Build history of the part. All positions in model axes, mm. Face numbers are marked on the shaded views. A direction names the side the tool comes from. Coordinates: 2 decimals unless noted, no trailing zeros. Loops run counter-clockwise (first coordinate to the right, second up) from the corner with the lowest first, then second, coordinate; pieces in that order, holes last.
(1) Slice it at A-A (y = 8). Give the cut face in (x, z).
(2) Slice it at D-D (z = 12.5). Give the number of separate pieces and of enclosed holes in the cut face, and give its area (3 significant figures).
(3) Wall check: L1, parallel to Y at x = -55, z = 11.75; L2, parallel to X at y = -48.5, z = 11.25; L3, parallel to X at y = 21.5, z = 11.75. Give the ranges that are in metal, low to high.
(4) Tool access for the marked faces 1 and 2: list every direction of +Z, -Z, +X, -X, +Y, -Y with a clear straight run to the whole face (end or side of a thin tool).
(5) Slice it at C-C (z = 18). Give the cut face in (x, y), and give its area (3 significant figures).
(6) Flat gauge pins, fed straight in: P1, Ø1.5, axis at y = 52.5, z = 7.5, coming from the -X side; P2, Ø1, axis at x = -56, y = -9, coming from the +Z side; P3, Ø3.5, axis at x = -89, z = 8.5, coming from the +Y side; P4, Ø4, axis at x = -59.61, y = -2.83, coming from the +Z side. Where does each tip first touch, or does it go through?
(7) Slice it at B-B (x = -77). Give the cut face in (y, z), and give its area (3 significant figures).
(8) Two-plate mould, pull along X, no slides. Class the marked faces 3, 4, 5 and 6: pulls with the +X half, pulls with the -X half, needs draft (parallel to the pull), parting line crosses it, or undercut.
from build123d import *

# Parameters (mm, degrees)
SALIENTE_EXTRUIR1_DEPTH      = 50
CROQUIS2_W                   = 40
CROQUIS2_H                   = 50
SALIENTE_EXTRUIR2_DEPTH      = 60
SALIENTE_EXTRUIR2_DEPTH_BACK = 31
REDONDEO1_R                  = 10
REDONDEO2_R                  = 10
CORTAR_EXTRUIR2_DEPTH        = 76
REDONDEO6_R                  = 5
VACIADO2_T                   = -3
CROQUIS4_R                   = 5
SALIENTE_EXTRUIR3_DEPTH      = 7
CROQUIS5_R                   = 2.5
CORTAR_EXTRUIR3_DEPTH        = 11
SALIENTE_EXTRUIR4_DEPTH      = 5
CROQUIS6_4_R                 = 2.5
CORTAR_EXTRUIR4_DEPTH        = 21
CORTAR_EXTRUIR7_REACH        = 62
CROQUIS8_R                   = 3.75
CORTAR_EXTRUIR8_REACH        = 64.5
CROQUIS9_W                   = 4
CROQUIS9_H                   = 8
CORTAR_EXTRUIR9_REACH        = 122
CROQUIS10_W                  = 10
CROQUIS10_H                  = 4


with BuildPart() as part:
    # Croquis1 → Saliente-Extruir1 (new body)
    with BuildSketch(Plane.XY):
        with BuildLine():
            Line((-80.606796451, 54.173553719), (-40.606796451, 54.173553719))
            ThreePointArc((-40.606796451, 54.173553719), (-33.53572864, 51.244621531), (-30.606796451, 44.173553719))
            Line((-30.606796451, 44.173553719), (-30.606796451, 4.173553719))
            ThreePointArc((-30.606796451, 4.173553719), (-33.53572864, -2.897514093), (-40.606796451, -5.826446281))
            Line((-40.606796451, -5.826446281), (-80.606796451, -5.826446281))
            ThreePointArc((-80.606796451, -5.826446281), (-87.677864263, -2.897514093), (-90.606796451, 4.173553719))
            Line((-90.606796451, 4.173553719), (-90.606796451, 44.173553719))
            ThreePointArc((-90.606796451, 44.173553719), (-87.677864263, 51.244621531), (-80.606796451, 54.173553719))
        make_face()
    extrude(amount=SALIENTE_EXTRUIR1_DEPTH)

    # Croquis2 → Saliente-Extruir2 (add, two sides)
    with BuildSketch(Plane.XZ.offset(5.826446281)) as saliente_extruir2_sk:
        with Locations((-50.606796451, 25)):
            Rectangle(CROQUIS2_W, CROQUIS2_H)
    extrude(amount=SALIENTE_EXTRUIR2_DEPTH)
    extrude(saliente_extruir2_sk.sketch, amount=-SALIENTE_EXTRUIR2_DEPTH_BACK)

    # Redondeo1
    redondeo1_edges = [part.edges().sort_by_distance(p)[0] for p in [
        (-30.606796451, -65.826446281, 25),
    ]]
    fillet(redondeo1_edges, radius=REDONDEO1_R)

    # Redondeo2
    redondeo2_edges = [part.edges().sort_by_distance(p)[0] for p in [
        (-70.606796451, -65.826446281, 25),
    ]]
    fillet(redondeo2_edges, radius=REDONDEO2_R)

    # Croquis3 → Cortar-Extruir2 (cut)
    with BuildSketch(Plane(origin=(-30.606796451, 0, 0), x_dir=(0, 0, -1), z_dir=(1, 0, 0))):
        Polygon((-20, -55.826446281), (-20, 57.222275959), (-50, 57.222275959), (-50, -55.826446281), (-50, -71.304791729), (-20, -71.304791729), align=None)
    extrude(amount=-CORTAR_EXTRUIR2_DEPTH, mode=Mode.SUBTRACT)

    # Redondeo6
    redondeo6_edges = [part.edges().sort_by_distance(p)[0] for p in [
        (-70.606796451, -5.826446281, 10),
    ]]
    fillet(redondeo6_edges, radius=REDONDEO6_R)

    # Vaciado2
    vaciado2_openings = [part.faces().sort_by_distance(p)[0] for p in [
        (-63.60975761, -5.496074106, 20),
    ]]
    offset(amount=VACIADO2_T, openings=vaciado2_openings, kind=Kind.INTERSECTION)

    # Croquis4 → Saliente-Extruir3 (add)
    with BuildSketch(Plane.XY.offset(3)):
        with Locations((-39.606796451, -2.826446281)):
            Circle(CROQUIS4_R)
        with Locations((-59.606796451, -2.826446281)):
            Circle(CROQUIS4_R)
    extrude(amount=SALIENTE_EXTRUIR3_DEPTH)

    # Croquis5 → Cortar-Extruir3 (cut, through all)
    with BuildSketch(Plane.XY.offset(10)):
        with Locations((-59.606796451, -2.826446281)):
            Circle(CROQUIS5_R)
        with Locations((-39.606796451, -2.826446281)):
            Circle(CROQUIS5_R)
    extrude(amount=-CORTAR_EXTRUIR3_DEPTH, mode=Mode.SUBTRACT)

    # Croquis6 → Saliente-Extruir4 (add)
    with BuildSketch(Plane.XY.offset(20)):
        with BuildLine():
            Line((-35.560225021, 61.520617947), (-48.606796451, 54.173553719))
            Line((-48.606796451, 54.173553719), (-40.606796451, 54.173553719))
            ThreePointArc((-40.606796451, 54.173553719), (-33.53572864, 51.244621531), (-30.606796451, 44.173553719))
            Line((-30.606796451, 44.173553719), (-30.606796451, 36.173553719))
            Line((-30.606796451, 36.173553719), (-28.142904197, 56.564123399))
            ThreePointArc((-28.142904197, 56.564123399), (-30.328790596, 61.321179473), (-35.560225021, 61.520617947))
        make_face()
    extrude(amount=-SALIENTE_EXTRUIR4_DEPTH)

    # Croquis6_4 → Cortar-Extruir4 (cut, through all)
    with BuildSketch(Plane.XY.offset(20)):
        with Locations((-33.106796451, 57.163934776)):
            Circle(CROQUIS6_4_R)
    extrude(amount=-CORTAR_EXTRUIR4_DEPTH, mode=Mode.SUBTRACT)

    # Croquis8 → Cortar-Extruir7 (cut, up to next)
    with BuildSketch(Plane(origin=(-30.606796451, 0, 0), x_dir=(0, 0, -1), z_dir=(1, 0, 0)), mode=Mode.PRIVATE) as cortar_extruir7_sk1:
        with Locations((-10.615433885, 29.173553719)):
            Circle(CROQUIS8_R)
    cortar_extruir7_tool1 = extrude(cortar_extruir7_sk1.sketch, amount=-CORTAR_EXTRUIR7_REACH, mode=Mode.PRIVATE) & part.part
    add(cortar_extruir7_tool1.solids().sort_by_distance((-30.606796, 29.173554, 10.615434))[0], mode=Mode.SUBTRACT)
    # Croquis8 → Cortar-Extruir7 (cut, up to next)
    with BuildSketch(Plane(origin=(-30.606796451, 0, 0), x_dir=(0, 0, -1), z_dir=(1, 0, 0)), mode=Mode.PRIVATE) as cortar_extruir7_sk2:
        with Locations((-10.615433885, 14.173553719)):
            Circle(CROQUIS8_R)
    cortar_extruir7_tool2 = extrude(cortar_extruir7_sk2.sketch, amount=-CORTAR_EXTRUIR7_REACH, mode=Mode.PRIVATE) & part.part
    add(cortar_extruir7_tool2.solids().sort_by_distance((-30.606796, 14.173554, 10.615434))[0], mode=Mode.SUBTRACT)
    # Croquis8 → Cortar-Extruir7 (cut, up to next)
    with BuildSketch(Plane(origin=(-30.606796451, 0, 0), x_dir=(0, 0, -1), z_dir=(1, 0, 0)), mode=Mode.PRIVATE) as cortar_extruir7_sk3:
        with Locations((-10.615433885, -0.826446281)):
            Circle(CROQUIS8_R)
    cortar_extruir7_tool3 = extrude(cortar_extruir7_sk3.sketch, amount=-CORTAR_EXTRUIR7_REACH, mode=Mode.PRIVATE) & part.part
    add(cortar_extruir7_tool3.solids().sort_by_distance((-30.606796, -0.826446, 10.615434))[0], mode=Mode.SUBTRACT)

    # Croquis9 → Cortar-Extruir8 (cut, up to next)
    with BuildSketch(Plane.ZY.offset(90.606796451), mode=Mode.PRIVATE) as cortar_extruir8_sk1:
        with Locations((9, 24.173553719)):
            Rectangle(CROQUIS9_W, CROQUIS9_H)
    cortar_extruir8_tool1 = extrude(cortar_extruir8_sk1.sketch, amount=-CORTAR_EXTRUIR8_REACH, mode=Mode.PRIVATE) & part.part
    add(cortar_extruir8_tool1.solids().sort_by_distance((-90.606796, 24.173554, 9))[0], mode=Mode.SUBTRACT)

    # Croquis10 → Cortar-Extruir9 (cut, up to next)
    with BuildSketch(Plane(origin=(0, 54.173553719, 0), x_dir=(1, 0, 0), z_dir=(0, 1, 0)), mode=Mode.PRIVATE) as cortar_extruir9_sk1:
        with Locations((-60.606796451, -7)):
            Rectangle(CROQUIS10_W, CROQUIS10_H)
    cortar_extruir9_tool1 = extrude(cortar_extruir9_sk1.sketch, amount=-CORTAR_EXTRUIR9_REACH, mode=Mode.PRIVATE) & part.part
    add(cortar_extruir9_tool1.solids().sort_by_distance((-60.606796, 54.173554, 7))[0], mode=Mode.SUBTRACT)


solid = part.part
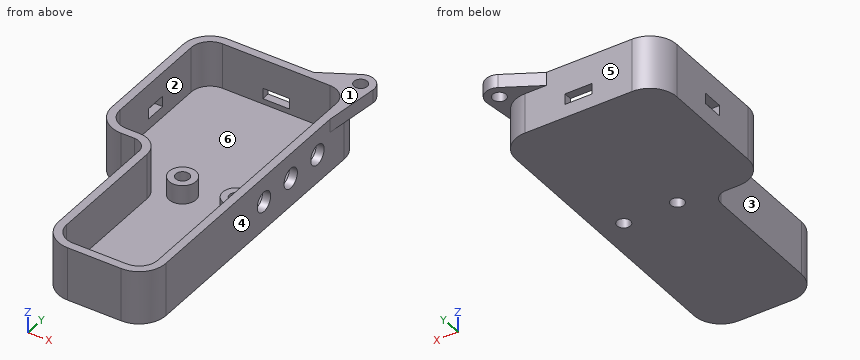
Response values:
1. outline: (-90.61, 0) - (-30.61, 0) - (-30.61, 20) - (-33.61, 20) - (-33.61, 3) - (-87.61, 3) - (-87.61, 20) - (-90.61, 20) - close
2. separate pieces: 3
2. enclosed holes: 0
2. area: 923 mm2
3. L1: y = -65.83 to -62.83, 51.17 to 54.17
3. L2: x = -70.61 to -67.61, -33.61 to -30.61
3. L3: x = -90.61 to -87.61, -33.61 to -30.61
4. face 1: +Z, +X, -X, +Y, -Y
4. face 2: +Z
5. outline: (-90.61, 4.17) arc R10 ccw to (-80.61, -5.83) - (-75.61, -5.83) arc R5 cw to (-70.61, -10.83) - (-70.61, -55.83) arc R10 ccw to (-60.61, -65.83) - (-40.61, -65.83) arc R10 ccw to (-30.61, -55.83) - (-30.61, 36.17) - (-28.14, 56.56) arc R5 ccw to (-35.56, 61.52) - (-48.61, 54.17) - (-80.61, 54.17) arc R10 ccw to (-90.61, 44.17) - close; hole (-87.61, 4.17) arc R7 ccw to (-80.61, -2.83) - (-75.61, -2.83) arc R8 cw to (-67.61, -10.83) - (-67.61, -55.83) arc R7 ccw to (-60.61, -62.83) - (-40.61, -62.83) arc R7 ccw to (-33.61, -55.83) - (-33.61, 44.17) arc R7 ccw to (-40.61, 51.17) - (-80.61, 51.17) arc R7 ccw to (-87.61, 44.17) - close; hole circle Ø5 at (-33.11, 57.16)
5. area: 1,100 mm2
6. P1: stops at x = -87.13
6. P2: stops at z = 3
6. P3: stops at y = 51.65
6. P4: passes through
7. outline: (-5.83, 0) - (54.17, 0) - (54.17, 20) - (51.17, 20) - (51.17, 3) - (-2.83, 3) - (-2.83, 20) - (-5.83, 20) - close
7. area: 282 mm2
8. face 3: pulls with the -X half
8. face 4: pulls with the +X half
8. face 5: needs draft
8. face 6: undercut
